from build123d import *

# Parameters (mm, degrees)
F0_W     = 35
F0_H     = 35
F1_DEPTH = 35
F2_R     = 17
F5_DEPTH = 35.001
F6_R     = 2


with BuildPart() as f1:
    # F0 (on Top) → F1 (new body)
    with BuildSketch(Plane.XY):
        Rectangle(F0_W, F0_H)
    extrude(amount=F1_DEPTH)

    # F2
    f2_edges = [f1.edges().sort_by_distance(p)[0] for p in [
        (0, -17.5, 35),
        (0, 17.5, 35),
    ]]
    fillet(f2_edges, radius=F2_R)

    # F4 (on face) → F5 (cut, through all)
    with BuildSketch(Plane.YZ.offset(17.5)):
        with BuildLine():
            ThreePointArc((17.5, 18), (16.7637891964, 22.9486524402), (14.6189222384, 27.4686870699))
            Line((14.6189222384, 27.4686870699), (-0.8730111465, 23.4686870699))
            ThreePointArc((-0.8730111465, 23.4686870699), (-4.8066349175, 16.7018804151), (2.0080666152, 12.8518270003))
            Line((2.0080666152, 12.8518270003), (17.5, 16.8518270003))
            Line((17.5, 16.8518270003), (17.5, 18))
        make_face()
    extrude(amount=-F5_DEPTH, mode=Mode.SUBTRACT)

    # F6
    f6_edges = [f1.edges().sort_by_distance(p)[0] for p in [
        (17.5, -17.5, 9),
        (17.5, 0, 0),
        (17.5, 17.5, 8.425914),
        (17.5, 9.754033, 14.851827),
        (17.5, -4.806635, 16.70188),
        (17.5, 6.872956, 25.468687),
        (17.5, 8.50101, 32.999461),
        (17.5, 0, 35),
        (17.5, -12.520815, 30.020815),
        (-17.5, 0, 0),
        (-17.5, -17.5, 9),
        (-17.5, -12.520815, 30.020815),
        (-17.5, 0, 35),
        (-17.5, 8.50101, 32.999461),
        (-17.5, 6.872956, 25.468687),
        (-17.5, -4.806635, 16.70188),
        (-17.5, 9.754033, 14.851827),
        (-17.5, 17.5, 8.425914),
        (0, 17.5, 16.851827),
        (0, 14.618922, 27.468687),
    ]]
    fillet(f6_edges, radius=F6_R)


solid = f1.part
Geometry check sheet. Reference: the model listing, model coordinates, mm. A direction names the side the tool comes from. Round coordinates to 2 decimals unless told otherwise and drop trailing zeros. Write each loop counter-clockwise with the first axis right and the second up, starting at its lowest first coordinate (ties: lowest second). Pieces come first, ordered by that corner, then holes. Notation, with made-up numbers: (-18.75, -29) - (19.25, -29) arc R13 cw to (19.25, -6) - close; hole circle Ø7 at (11.25, 12). An arc over 180 degrees is marked (long way). One line per item, written item: value.
1. Set-up check for faces 1 (the face through (16.9, 5.1, 25.6)), 2 (the face through (-16.93, 5.295, 25.683)), 3 (the face through (16.9, 8.74, 14)): record each of +Z, -Z, +X, -X, +Y, -Y from which the full face is reachable in a straight line by a thin tool's end or side.
The answers:
face 1: +X, +Y
face 2: -X, +Y
face 3: +X
2. Depth check by flat-ended pin: pin 1 Ø12 at (x, z) = (-9, 21.5) entering from -Y; pin 2 Ø6 at (x, z) = (11.5, 28) entering from -Y. Enter the tip coordinate at first touch or a pass-through.
The answers:
pin 1: stops at y = -17.5
pin 2: stops at y = -15.99
3. Cross-section at A-A on x = 5. Record the boundary of the cut face in (y, z), and give its area (3 significant figures).
The answers:
outline: (-17.5, 0) - (17.5, 0) - (17.5, 14.27) arc R2 ccw to (15, 16.21) - (2.01, 12.85) arc R5.5 cw (long way) to (-0.87, 23.47) - (11.59, 26.69) arc R2 ccw to (12.5, 30.04) arc R17 ccw to (0.5, 35) - (-0.5, 35) arc R17 ccw to (-17.5, 18) - close
area: 866 mm^2
4. Scan lines: L1, parallel to Z at x = -1, y = 8; L2, parallel to Z at x = 4, y = 10.5; L3, parallel to X at y = 5, z = 33.5. Record each from-to range of solid material in increasing order.
The answers:
L1: z = 0 to 14.4, 25.76 to 33.26
L2: z = 0 to 15.04, 26.41 to 31.75
L3: x = -17.14 to 17.14
5. Mould release check, pull along Y, two halves, no side actions. Record for faces 4 (the face through (0, 17.5, 7)), 5 (the face through (-16.93, -16.9, 9.13)), 6 (the face through (0.217, 8.413, 14.506)): released by +Y, released by -Y, zero draft, split by the parting line, or undercut.
The answers:
face 4: released by +Y
face 5: released by -Y
face 6: undercut
